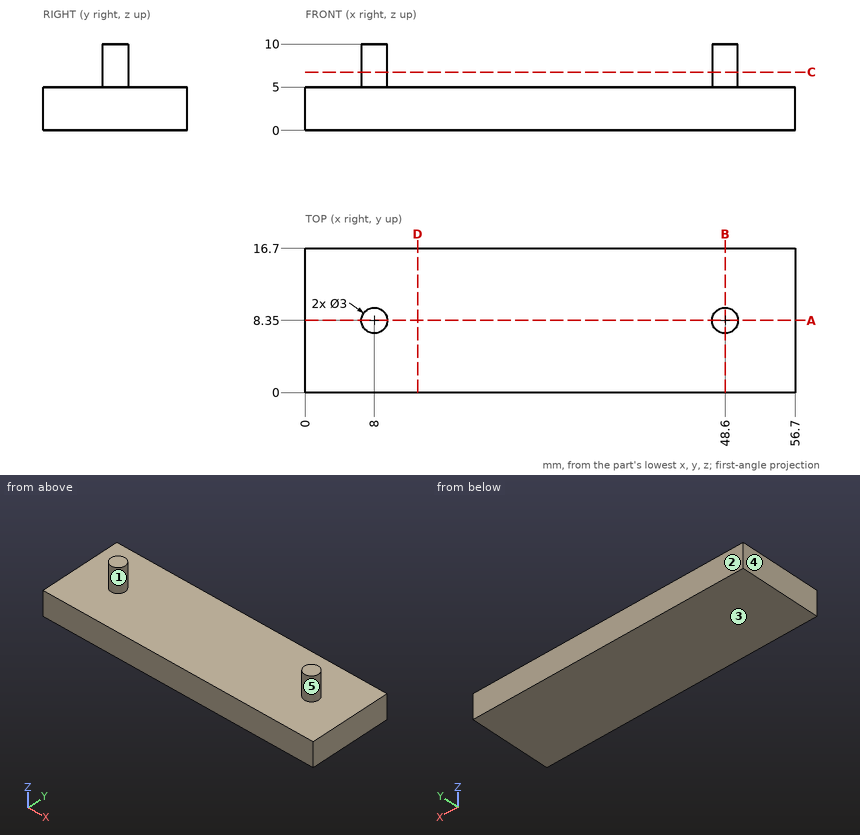
Check sheet for the drawn part. Datum: minimum x, y, z corner. Units: mm. A direction names the side the tool comes from. Round coordinates to 2 decimals unless told otherwise and drop trailing zeros. Write each loop counter-clockwise with the first axis right and the second up, starting at its lowest first coordinate (ties: lowest second). Pieces come first, ordered by that corner, then holes. Notation, with made-up numbers: (5.25, 85) -> (60.25, 85) arc R30 ccw to (60.25, 123) -> close; hole circle Ø7 at (-7, -39). An arc over 180 degrees is marked (long way). Put each result on its own line as item: value.
(1) Sectioned sample at C-C (z = 6.75). Enter the section's corners in (x, y), plus the area to 3 significant figures.
Values found:
outline: circle Ø3 at (8, 8.35); circle Ø3 at (48.6, 8.35)
area: 14.1 mm^2
(2) Material ranges on line 1 (Z direction, x = 12, y = 5.75); line 2 (X direction, y = 9, z = 7.5); line 3 (X direction, y = 9.25, z = 9), recorded low to high.
Values found:
line 1: z = 0 to 5
line 2: x = 6.65 to 9.35, 47.25 to 49.95
line 3: x = 6.8 to 9.2, 47.4 to 49.8
(3) Sectioned sample at D-D (x = 13). Enter the section's corners in (y, z).
Values found:
outline: (0, 0) -> (16.7, 0) -> (16.7, 5) -> (0, 5) -> close
(4) Sectioned sample at B-B (x = 48.6). Enter the section's corners in (y, z).
Values found:
outline: (0, 0) -> (16.7, 0) -> (16.7, 5) -> (9.85, 5) -> (9.85, 10) -> (6.85, 10) -> (6.85, 5) -> (0, 5) -> close
(5) Tool access check on the marked faces 1 and 2. Record the directions out of +Z, -Z, +X, -X, +Y, -Y that give a thin tool (end or side, any length) a straight path to the whole face; none if there is none.
Values found:
face 1: +Z
face 2: +Z, -Z, +X, -X, +Y
(6) Mould release check, pull along X, two halves, no side actions. Record for the marked faces 3, 4 and 5: released by +X, released by -X, zero draft, split by the parting line, or undercut.
Values found:
face 3: zero draft
face 4: released by -X
face 5: undercut
(7) Go/stop test with flat-tipped pins: pin 1 Ø2 at (x, y) = (7.5, 4.5) entering from -Z; pin 2 Ø5 at (x, y) = (41.5, 8.5) entering from +Z. Record where each tip stops, or that it passes through.
Values found:
pin 1: stops at z = 0
pin 2: stops at z = 5
(8) Sectioned sample at A-A (y = 8.35). Enter the section's corners in (x, z), plus the area to 4 significant figures.
Values found:
outline: (0, 0) -> (56.7, 0) -> (56.7, 5) -> (50.1, 5) -> (50.1, 10) -> (47.1, 10) -> (47.1, 5) -> (9.5, 5) -> (9.5, 10) -> (6.5, 10) -> (6.5, 5) -> (0, 5) -> close
area: 313.5 mm^2
